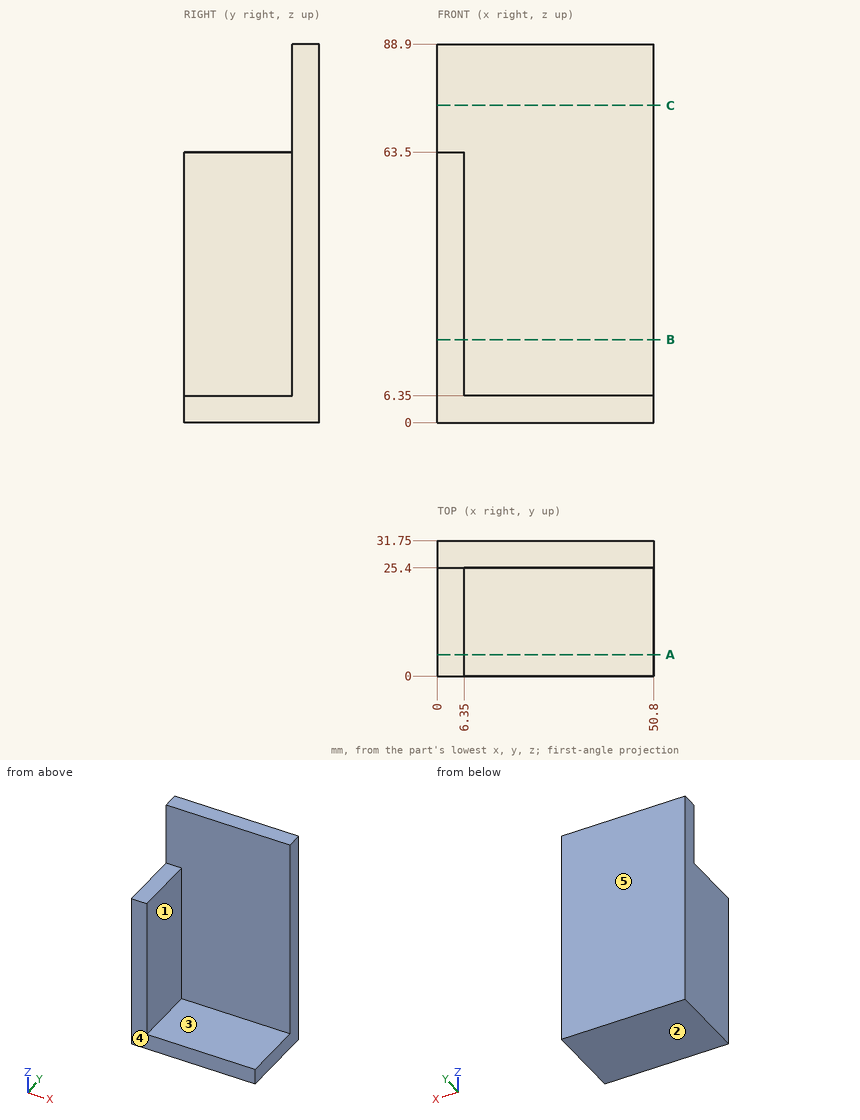
Geometry: see drawing. Coordinates: mm, zero at the bounding-box minimum. A direction names the side the tool comes from. Coordinates: 2 decimals unless noted, no trailing zeros. Order: outer loops, then holes, each group sorted by start corner. A loop starts at its lowest first (then second) coordinate and runs counter-clockwise, first axis right, second up. Notation, with made-up numbers: M 74,34.25 L 95,34.25 A28 ccw 95,54.25 Z; hole C 6,18.25 d10. An arc over 180 degrees is marked long. Write item = value, one per line. Start each with the question number.
(1) Section B-B on z = 19.5. Output: boundary loops of the cut face in (x, y), and give its area (3 significant figures).
(2) Section A-A on y = 5. Output: boundary loops of the cut face in (x, z), and give its area (3 significant figures).
(3) First-contact query: P1, Ø5, axis at x = 19, y = 18, coming from the +Z side; P2, Ø1, axis at y = 20.5, z = 36.5, coming from the +X side; P3, Ø1.5, axis at x = 8.5, z = 66.5, coming from the -Y side. Flat tips, straight axial feed; report the tip coordinate or a pass-through.
(4) Line query: line 1 along Y through (x, z) = (32, 59); line 2 along Z through (x, y) = (44, 23). Output: solid intervals per line, ascending. Write a range as [from, to].
(5) Section C-C on z = 74.5. Output: boundary loops of the cut face in (x, y).
(6) Reachability of the marked faces 1 and 2 from +Z, -Z, +X, -X, +Y, -Y: full face, straight path, thin tool, end or side. Return the list, or none.
(7) Pull-direction query (Y, two-part tool) for the marked faces 3, 4 and 5; classes: released by +Y, released by -Y, zero draft, split by the parting line, or undercut.
Result set:
q1.outline = M 0,0 L 6.35,0 L 6.35,25.4 L 50.8,25.4 L 50.8,31.75 L 0,31.75 Z
q1.area = 484 mm²
q2.outline = M 0,0 L 50.8,0 L 50.8,6.35 L 6.35,6.35 L 6.35,63.5 L 0,63.5 Z
q2.area = 685 mm²
q3.P1 = 6.35
q3.P2 = 6.35
q3.P3 = 25.4
q4.line_1 = [25.4, 31.75]
q4.line_2 = [0, 6.35]
q5.outline = M 0,25.4 L 50.8,25.4 L 50.8,31.75 L 0,31.75 Z
q6.face_1 = +Z, +X, -Y
q6.face_2 = -Z, +X, -X, +Y, -Y
q7.face_3 = zero draft
q7.face_4 = released by -Y
q7.face_5 = released by +Y
